Input: part model. Units: mm. Frame: model coordinates. Face numbers are marked on the shaded views. A direction names the side the tool comes from. Coordinates: 2 decimals unless noted, no trailing zeros. Loops run counter-clockwise (first coordinate to the right, second up) from the corner with the lowest first, then second, coordinate; pieces in that order, holes last. Notation, with made-up numbers: (52.25, 71.5) - (105.25, 71.5) arc R28 ccw to (105.25, 100.5) - close; hole circle Ø2 at (-14.5, 54.25). An arc over 180 degrees is marked (long way). Use a Markdown table: item, result. Add a question column.
1. Section query D-D on y = -12.45. Return the cut outline in (x, z) (3 decimals), then the cut area to 3 significant figures.
2. Draft query along X for the marked faces 3, 4 and 5. Return one class per face: released by +X, released by -X, zero draft, split by the parting line, or undercut.
3. Ray query, L1, parallel to Y at x = 1.5, z = 25.6; L2, parallel to Z at x = 0.7, y = -12.45; L3, parallel to Y at x = 7.6, z = 50.25. Return the intervals inside material, ascending. Write a range as [from, to].
4. Contact query for flat-ended pins moving along their axis: P1, Ø6, axis at x = 5.5, y = -30.5, coming from the +Z side; P2, Ø12, axis at x = 7.5, z = 18, coming from the -Y side; P3, Ø3.5, axis at x = 1, y = -25, coming from the +Z side; P4, Ø19, axis at y = -26, z = 20.5, coming from the -X side. Output: stop coordinate, or through.
5. Section query A-A on z = 2.6. Return the cut outline in (x, y) (3 decimals).
6. Section query B-B on x = 7.6. Return the cut outline in (y, z).
7. Section query C-C on y = -2.15. Return the cut outline in (x, z) (1 decimal), then the cut area to 3 significant figures.
8. Access query for the marked faces 1 and 2. Directions: +Z, -Z, +X, -X, +Y, -Y. A direction counts if a zero-diameter tool reaches every point of the face in a straight line with its end or side. Return the directions, or none.
Autodesk Inventor part; units mm, degrees
ref_plane "YZ Plane" through (0, 0, 0) normal (1, 0, 0) x (0, 1, 0)
ref_plane "XZ Plane" through (0, 0, 0) normal (0, 1, 0) x (-1, 0, 0)
ref_plane "XY Plane" through (0, 0, 0) normal (0, 0, 1) x (1, 0, 0)
sketch "Sketch1" plane through (0, 0, 0) normal (0, 0, 1) x (1, 0, 0)
  line L0 (0, 0) -> (0, -38.05)
  line L1 (0, -38.05) -> (3.175, -38.05)
  line L2 (3.175, -38.05) -> (3.175, 0)
  line L3 (3.175, 0) -> (0, 0)
  line L4 (3.175, 0) -> (3.175, -6.85)
  line L5 (3.175, -6.85) -> (12.025, -6.85)
  line L6 (12.025, -6.85) -> (12.025, 0)
  line L7 (12.025, 0) -> (15.2, 0)
  line L8 (15.2, 0) -> (15.2, -6.85)
  line L9 (15.2, -6.85) -> (15.2, -8.85)
  line L10 (15.2, -8.85) -> (3.175, -8.85)
  line L11 (0, -38.05) -> (0, -31.2)
  dimension "d0" = 38.05
  dimension "d1" = 3.175
  dimension "d2" = 6.85
  dimension "d3" = 8.85
  dimension "d4" = 3.175
  dimension "d5" = 2
extrude "Extrusion1" add sketch "Sketch1" along normal blind 49.213
sketch "Sketch2" plane through (0, 0, 0) normal (0, 0, -1) x (-1, 0, 0)
  line L0 (0, -38.05) -> (-3.175, -38.05)
  line L1 (0, -38.05) -> (0, -32.05)
  line L2 (0, 0) -> (0, -38.05)
  line L3 (0, -32.05) -> (0, -23.25)
  line L4 (0, -23.25) -> (6.6, -23.25)
  line L5 (6.6, -23.25) -> (6.6, -32.05)
  line L6 (6.6, -32.05) -> (0, -32.05)
  dimension "d12" = 6
  dimension "d13" = 8.8
  dimension "d14" = 6.6
extrude "Extrusion2" add sketch "Sketch2" against normal blind 3.175
sketch "Sketch3" plane through (0, 0, 3.175) normal (0, 0, 1) x (1, 0, 0)
  line L0 (0, -23.25) -> (0, -32.05)
  line L1 (0, -23.25) -> (-3.3, -23.25)
  line L2 (0, -23.25) -> (-6.6, -23.25)
  line L3 (-3.3, -23.25) -> (-3.3, -27.65)
  point P0 (0, 0)
  dimension "d17" = 4.4
hole "Hole1" at (-3.3, -27.65, 3.175) direction (0, 0, -1) diameter 3 end through all
fillet "Fillet1" radius 2 2 edges at (-6.6, -23.25, 1.5875) (-6.6, -32.05, 1.5875)
sketch "Sketch4" plane through (0, 0, 49.213) normal (0, 0, 1) x (1, 0, 0)
  line L0 (3.175, 0) -> (0, 0)
  line L1 (3.175, -8.85) -> (15.2, -8.85)
  line L2 (0, 0) -> (15.2, 0)
  line L3 (15.2, 0) -> (15.2, -8.85)
  line L4 (15.2, -8.85) -> (0, -8.85)
  line L5 (0, -8.85) -> (0, 0)
extrude "Extrusion3" add sketch "Sketch4" along normal blind 1.5875
sketch "Sketch5" plane through (0, 0, 50.8005) normal (0, 0, 1) x (1, 0, 0)
  line L0 (3.175, 0) -> (0, 0)
  line L1 (0, 0) -> (3.175, 0)
  line L2 (3.175, 0) -> (12.025, 0)
  line L3 (3.175, 0) -> (7.6, 0)
  line L4 (7.6, 0) -> (7.6, -3.425)
  dimension "d28" = 3.425
hole "Hole2" at (7.6, -3.425, 50.8005) direction (0, 0, -1) diameter 3 end through all
fillet "Fillet2" radius 2 2 edges at (0, -8.85, 50.0068) (15.2, -8.85, 25.4003)
sketch "Sketch6" plane through (0, -38.05, 0) normal (-1, 0, 0) x (0, 0, 1)
  line L0 (0, 0) -> (0, 29.2)
  line L1 (0, 0) -> (0, 28.2)
  line L2 (0, 28.2) -> (28.2, 28.2)
  line L3 (28.2, 28.2) -> (28.2, 0)
  line L4 (0, 0) -> (49.213, 0)
  line L5 (0, 0) -> (0, 14.1)
  line L6 (0, 12.8) -> (0, 14.8)
  line L7 (0, 14.1) -> (14.1, 14.1)
  line L8 (14.1, 14.1) -> (2.6, 14.1)
  line L9 (2.6, 14.1) -> (2.6, 2.6)
  line L10 (0, 12.8) -> (3.175, 12.8)
  line L11 (2.6, 2.6) -> (25.6, 2.6)
  line L12 (25.6, 2.6) -> (25.6, 25.6)
  line L13 (25.6, 25.6) -> (2.6, 25.6)
  line L14 (2.6, 25.6) -> (2.6, 2.6)
  point P0 (0, 38.05)
  dimension "d37" = 28.2
  dimension "d38" = 28.2
  dimension "d39" = 11.5
  dimension "d40" = 11.5
  dimension "d41" = 90
  dimension "d42" = 23
  dimension "d43" = 23
hole "Hole3" at (0, -35.45, 2.6) at (0, -35.45, 25.6) at (0, -12.45, 25.6) at (0, -12.45, 2.6) direction (1, 0, 0) diameter 2.5 end through all
delete faces "Delete1" heal yes whole lump no faces at (7.7207, -4.9201, 50.2713)
sketch "Sketch7" plane through (0, 0, 50.8005) normal (0, 0, 1) x (1, 0, 0)
  line L0 (15.2, -6.85) -> (15.2, 0)
  line L1 (15.2, 0) -> (0, 0)
  line L2 (15.2, 0) -> (0, 0)
  line L3 (0, 0) -> (7.6, 0)
  line L4 (7.6, 0) -> (7.6, -2.15)
  dimension "d51" = 2.15
hole "Hole4" at (7.6, -2.15, 50.8005) direction (0, 0, -1) diameter 3 depth 3.5
sketch "Sketch8" plane through (0, 0, 49.213) normal (0, 0, 1) x (1, 0, 0)
  line L0 (0, -38.05) -> (3.175, -38.05)
  line L1 (3.175, -38.05) -> (0, -38.05)
  line L2 (3.175, -23.45) -> (0, -23.45)
  line L3 (0, -23.45) -> (0, -17.45)
  line L4 (0, -17.45) -> (3.175, -17.45)
  line L5 (3.175, -17.45) -> (3.175, -23.45)
  line L6 (3.175, -23.45) -> (0, -23.45)
  line L7 (0, -23.45) -> (0, -29.45)
  line L8 (0, -29.45) -> (3.175, -29.45)
  line L9 (3.175, -29.45) -> (3.175, -23.45)
  point P0 (0, 0)
  point P1 (3.175, -8.85)
  dimension "d59" = 6
  dimension "d60" = 6
extrude "Extrusion4" cut sketch "Sketch8" against normal blind 3.175
fillet "Fillet3" radius 2 2 edges at (1.5875, -17.45, 46.038) (1.5875, -29.45, 46.038)
properties part number "Yaw Motor Mount"
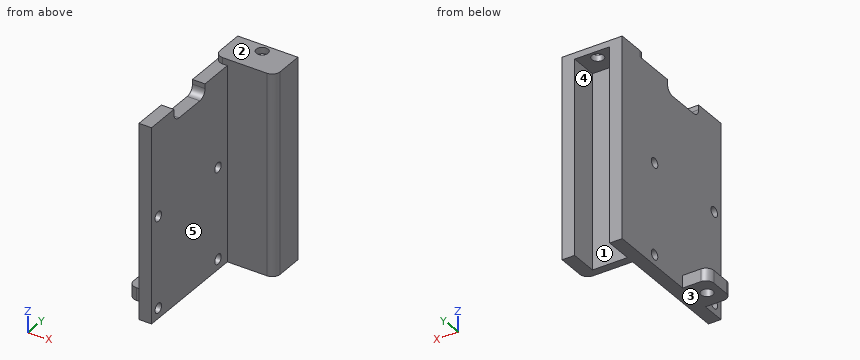
Resolved:
| question | item | result |
|---|---|---|
| 1 | outline | (0, 0) - (3.175, 0) - (3.175, 1.35) - (0, 1.35) - close; (0, 3.85) - (3.175, 3.85) - (3.175, 24.35) - (0, 24.35) - close; (0, 26.85) - (3.175, 26.85) - (3.175, 49.213) - (0, 49.213) - close |
| 1 | area | 140 mm² |
| 2 | face 3 | zero draft |
| 2 | face 4 | undercut |
| 2 | face 5 | released by +X |
| 3 | L1 | [-38.05, -36.7], [-34.2, -13.7], [-11.2, 0] |
| 3 | L2 | [0, 1.35], [3.85, 24.35], [26.85, 49.21] |
| 3 | L3 | [-8.85, -3.65], [-0.65, 0] |
| 4 | P1 | z = 49.21 |
| 4 | P2 | y = -38.05 |
| 4 | P3 | z = 46.04 |
| 4 | P4 | x = 0 |
| 5 | outline | (-6.6, -30.05) arc R2 ccw to (-4.6, -32.05) - (0, -32.05) - (0, -34.2) - (3.175, -34.2) - (3.175, -13.7) - (0, -13.7) - (0, -23.25) - (-4.6, -23.25) arc R2 ccw to (-6.6, -25.25) - close; (0, -38.05) - (3.175, -38.05) - (3.175, -36.7) - (0, -36.7) - close; (0, -11.2) - (3.175, -11.2) - (3.175, -8.85) - (13.2, -8.85) arc R2 ccw to (15.2, -6.85) - (15.2, 0) - (12.025, 0) - (12.025, -6.85) - (3.175, -6.85) - (3.175, 0) - (0, 0) - close; hole circle Ø3 at (-3.3, -27.65) |
| 6 | outline | (-8.85, 0) - (-6.85, 0) - (-6.85, 49.21) - (-3.65, 49.21) - (-3.65, 50.8) - (-8.85, 50.8) - close; (-0.65, 49.21) - (0, 49.21) - (0, 50.8) - (-0.65, 50.8) - close |
| 7 | outline | (0, 0) - (3.2, 0) - (3.2, 49.2) - (6.1, 49.2) - (6.1, 50.8) - (0, 50.8) - close; (9.1, 49.2) - (12, 49.2) - (12, 0) - (15.2, 0) - (15.2, 50.8) - (9.1, 50.8) - close |
| 7 | area | 332 mm² |
| 8 | face 1 | -Z, +Y |
| 8 | face 2 | +Z, +X, -X, +Y, -Y |
